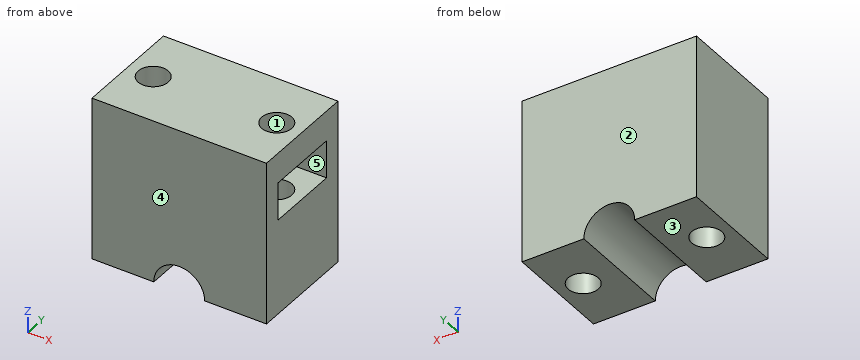
from build123d import *

# Parameters (mm, degrees)
SKETCH1_W               = 48
SKETCH1_H               = 45
BOSS_EXTRUDE1_DEPTH     = 30
SKETCH2_W               = 10.4
SKETCH2_H               = 20.4
CUT_EXTRUDE1_DEPTH      = 45
SKETCH3_R               = 4.15
CUT_EXTRUDE2_DEPTH      = 46
CUT_EXTRUDE3_DEPTH      = 1
CUT_EXTRUDE3_DEPTH_BACK = 31


with BuildPart() as part:
    # Sketch1 → Boss-Extrude1 (new body)
    with BuildSketch(Plane(origin=(0, 0, 0), x_dir=(1, 0, 0), z_dir=(0, 1, 0))):
        Rectangle(SKETCH1_W, SKETCH1_H)
    extrude(amount=BOSS_EXTRUDE1_DEPTH)

    # Sketch2 → Cut-Extrude1 (cut)
    with BuildSketch(Plane(origin=(24, 0, 0), x_dir=(0, 0, -1), z_dir=(1, 0, 0))):
        with Locations((-9, 15)):
            Rectangle(SKETCH2_W, SKETCH2_H)
    extrude(amount=-CUT_EXTRUDE1_DEPTH, mode=Mode.SUBTRACT)

    # Sketch3 → Cut-Extrude2 (cut, through all)
    with BuildSketch(Plane.XY.offset(22.5)):
        with Locations((-17, 15)):
            Circle(SKETCH3_R)
        with Locations((17, 15)):
            Circle(SKETCH3_R)
    extrude(amount=-CUT_EXTRUDE2_DEPTH, mode=Mode.SUBTRACT)

    # Sketch4 → Cut-Extrude3 (cut, two sides)
    with BuildSketch(Plane(origin=(0, 30, 0), x_dir=(1, 0, 0), z_dir=(0, 1, 0))) as cut_extrude3_sk:
        with BuildLine():
            Line((-7, 141.788608739), (-7, 22.5))
            ThreePointArc((-7, 22.5), (0, 15.5), (7, 22.5))
            Line((7, 22.5), (7, 141.788608739))
            Line((7, 141.788608739), (7, 380.365826216))
            Line((7, 380.365826216), (-7, 380.365826216))
            Line((-7, 380.365826216), (-7, 141.788608739))
        make_face()
    extrude(amount=CUT_EXTRUDE3_DEPTH, mode=Mode.SUBTRACT)
    extrude(cut_extrude3_sk.sketch, amount=-CUT_EXTRUDE3_DEPTH_BACK, mode=Mode.SUBTRACT)


solid = part.part
Could you check a few things on this model? Use its own coordinates, in mm. Face numbers are marked on the shaded views. A direction names the side the tool comes from. Coordinates: 2 decimals unless noted, no trailing zeros. Loops run counter-clockwise (first coordinate to the right, second up) from the corner with the lowest first, then second, coordinate; pieces in that order, holes last.
1. Imagine slicing it at B-B (y = 15). Please give me the cut outline in (x, z).
2. For P1, Ø3, axis at x = -7.5, z = 3, coming from the -Y side; P2, Ø5, axis at x = 17, y = 15, coming from the -Z side, each with a flat end and sliding along its axis, tell me the tip position at first contact or that it passes through.
3. Imagine slicing it at D-D (x = 15). Please give me the cut outline in (y, z).
4. I need wall thicknesses on L1, parallel to Y at x = 17, z = 17; L2, parallel to Y at x = 21, z = 7; L3, parallel to Z at x = -16, y = 10.5. Which ranges of each line are inside material? Lowest first, please.
5. We'd pull the mould along Y, two halves only. Please class the marked faces 1, 2 and 3: released by +Y, released by -Y, zero draft, split by the parting line, or undercut.
6. For the marked faces 4 and 5, which set-ups out of +Z, -Z, +X, -X, +Y, -Y let a thin tool reach every point of the face, with its end or its side?
7. Imagine slicing it at A-A (x = 8.5). Please give me the cut outline in (y, z), and give its area (3 significant figures).
8. Imagine slicing it at C-C (z = -11). Please give me the cut outline in (x, y).
Computed values:
1. outline: (-24, -22.5) - (-21.15, -22.5) - (-21.15, 22.5) - (-24, 22.5) - close; (-12.85, -22.5) - (-7, -22.5) arc R7 cw to (7, -22.5) - (12.85, -22.5) - (12.85, 3.8) - (-12.85, 3.8) - close; (-12.85, 14.2) - (12.85, 14.2) - (12.85, 22.5) - (-12.85, 22.5) - close; (21.15, -22.5) - (24, -22.5) - (24, 3.8) - (21.15, 3.8) - close; (21.15, 14.2) - (24, 14.2) - (24, 22.5) - (21.15, 22.5) - close
2. P1: stops at y = 0
2. P2: passes through
3. outline: (0, -22.5) - (11.36, -22.5) - (11.36, 3.8) - (4.8, 3.8) - (4.8, 14.2) - (11.36, 14.2) - (11.36, 22.5) - (0, 22.5) - close; (18.64, -22.5) - (30, -22.5) - (30, 22.5) - (18.64, 22.5) - (18.64, 14.2) - (25.2, 14.2) - (25.2, 3.8) - (18.64, 3.8) - close
4. L1: y = 0 to 10.85, 19.15 to 30
4. L2: y = 0 to 4.8, 25.2 to 30
4. L3: z = -22.5 to 3.8, 14.2 to 22.5
5. face 1: undercut
5. face 2: released by +Y
5. face 3: zero draft
6. face 4: +Z, -Z, +X, -X, -Y
6. face 5: +X
7. outline: (0, -22.5) - (30, -22.5) - (30, 22.5) - (0, 22.5) - close; hole (4.8, 3.8) - (25.2, 3.8) - (25.2, 14.2) - (4.8, 14.2) - close
7. area: 1,140 mm2
8. outline: (-24, 0) - (24, 0) - (24, 30) - (-24, 30) - close; hole circle Ø8.3 at (-17, 15); hole circle Ø8.3 at (17, 15)
